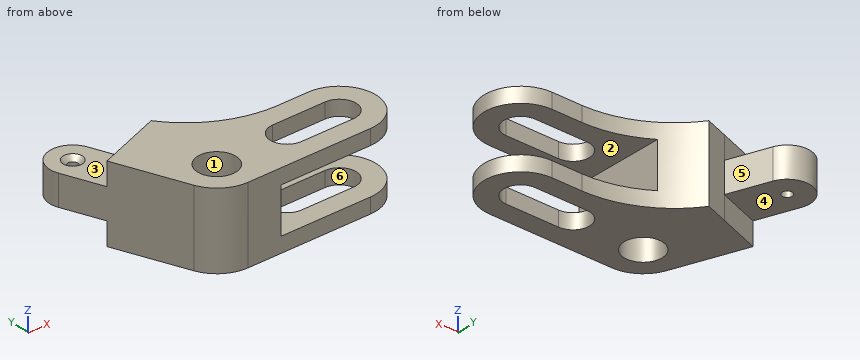
```python
from build123d import *

# Parameters (mm, degrees)
SKETCH1_R                                       = 12.5
SKETCH1_R_2                                     = 3
BOSS_EXTRUDE1_DEPTH                             = 25
SKETCH2_W                                       = 15
SKETCH2_H                                       = 43
CUT_EXTRUDE1_DEPTH                              = 50
CUT_EXTRUDE2_DEPTH                              = 125.934480099
CUT_EXTRUDE2_DEPTH_BACK                         = 125.934480099
SKETCH4_W                                       = 100
SKETCH4_H                                       = 30
CSK_FOR_M6_FLAT_HEAD_MACHINE_SCREW1_D           = 6.6
CSK_FOR_M6_FLAT_HEAD_MACHINE_SCREW1_CSINK_D     = 12.6
CSK_FOR_M6_FLAT_HEAD_MACHINE_SCREW1_CSINK_ANGLE = 90


with BuildPart() as part:
    # Sketch1 → Boss-Extrude1 (new, symmetric)
    with BuildSketch(Plane.XY):
        with BuildLine():
            Line((0, -24), (82, -24))
            ThreePointArc((82, -24), (106, 0), (82, 24))
            Line((82, 24), (62, 24))
            ThreePointArc((62, 24), (29.043180304, 32.086461832), (3.572230491, 54.509074192))
            Line((3.572230491, 54.509074192), (-11.462851442, 49.036751899))
            Line((-11.462851442, 49.036751899), (-21.039415455, 75.348145281))
            ThreePointArc((-21.039415455, 75.348145281), (-40.265106916, 84.313232443), (-49.230194078, 65.087540981))
            Line((-49.230194078, 65.087540981), (-39.653630065, 38.776147599))
            Line((-39.653630065, 38.776147599), (-22.552622899, -8.20848344))
            ThreePointArc((-22.552622899, -8.20848344), (-13.765834472, -19.659649063), (0, -24))
        make_face()
        Circle(SKETCH1_R, mode=Mode.SUBTRACT)
        with Locations((-35.134804766, 70.217843131)):
            Circle(SKETCH1_R_2, mode=Mode.SUBTRACT)
        with BuildLine():
            Line((47, 11), (82, 11))
            ThreePointArc((82, 11), (93, 0), (82, -11))
            Line((82, -11), (47, -11))
            ThreePointArc((47, -11), (36, 0), (47, 11))
        make_face(mode=Mode.SUBTRACT)
    extrude(amount=BOSS_EXTRUDE1_DEPTH, both=True)

    # Sketch2 → Cut-Extrude1 (cut)
    with BuildSketch(Plane(origin=(5.638155725, 2.05212086, 0), x_dir=(0, 0, -1), z_dir=(0.9396926207859104, 0.3420201433256632, 0))):
        with Locations((-17.5, 71.5)):
            Rectangle(SKETCH2_W, SKETCH2_H)
        with Locations((17.5, 71.5)):
            Rectangle(SKETCH2_W, SKETCH2_H)
    extrude(amount=-CUT_EXTRUDE1_DEPTH, mode=Mode.SUBTRACT)

    # Sketch4 → Cut-Extrude2 (cut, two sides: drawn at the far end of the back side and taken through both)
    with BuildSketch(Plane(origin=(0, 24, 0), x_dir=(1, 0, 0), z_dir=(0, 1, 0)).offset(-CUT_EXTRUDE2_DEPTH_BACK)):
        with Locations((72, 0)):
            Rectangle(SKETCH4_W, SKETCH4_H)
    extrude(amount=CUT_EXTRUDE2_DEPTH + CUT_EXTRUDE2_DEPTH_BACK, mode=Mode.SUBTRACT)

    # CSK for M6 Flat Head Machine Screw1 (through all)
    with Locations(Plane.XY.offset(10)):
        with Locations((-35.134804766, 70.217843131)):
            CounterSinkHole(CSK_FOR_M6_FLAT_HEAD_MACHINE_SCREW1_D / 2, CSK_FOR_M6_FLAT_HEAD_MACHINE_SCREW1_CSINK_D / 2, counter_sink_angle=CSK_FOR_M6_FLAT_HEAD_MACHINE_SCREW1_CSINK_ANGLE)


solid = part.part
```
The listing builds one solid part. Answer for the finished solid, in the listing's coordinates (mm). Face numbers are marked on the shaded views. A direction names the side the tool comes from. Round coordinates to 2 decimals unless told otherwise and drop trailing zeros. Write each loop counter-clockwise with the first axis right and the second up, starting at its lowest first coordinate (ties: lowest second). Pieces come first, ordered by that corner, then holes. Notation, with made-up numbers: (-4, -12) -> (7, -12) arc R12 cw to (7, 2) -> close; hole circle Ø6 at (69.25, 36). An arc over 180 degrees is marked (long way). Write item = value, one per line.
1) Which of the six approach directions +Z, -Z, +X, -X, +Y, -Y give full straight-line access (tool end or side, diameter ignored) to the marked faces 4, 5 and 6?
Check values:
face_4 = -Z, -X, +Y
face_5 = +Z, -Z, +Y
face_6 = +Z, -Z
2) Section D-D on x = 32.5 is taken. Write down the section's boundary in (y, z), plus the area to 3 significant figures.
Check values:
outline = (-24, -25) -> (30.4, -25) -> (30.4, -15) -> (-24, -15) -> close; (-24, 15) -> (30.4, 15) -> (30.4, 25) -> (-24, 25) -> close
area = 1,090 mm²
3) Section A-A on x = 77.5 is taken. Write down the section's boundary in (y, z).
Check values:
outline = (-24, -25) -> (-11, -25) -> (-11, -15) -> (-24, -15) -> close; (-24, 15) -> (-11, 15) -> (-11, 25) -> (-24, 25) -> close; (11, -25) -> (24, -25) -> (24, -15) -> (11, -15) -> close; (11, 15) -> (24, 15) -> (24, 25) -> (11, 25) -> close
4) For a pull along Z with two mould halves and no side action, classify the marked faces 1, 2 and 3 as released by +Z, released by -Z, zero draft, split by the parting line, or undercut.
Check values:
face_1 = zero draft
face_2 = undercut
face_3 = released by +Z
5) Straight lines are drawn through the part: line 1 along Z through (x, y) = (35.5, 8); line 2 along X through (y, z) = (4, -17); line 3 along Y through (x, z) = (0, 3). For each, find the intervals that lie inside material, in ascending order. Write a range as [from, to].
Check values:
line_1 = [-25, -15], [15, 25]
line_2 = [-27, -11.84], [11.84, 36.75], [92.25, 105.66]
line_3 = [-24, -12.5], [12.5, 53.21]
6) Given pin 1 (1 mm diameter, centred on x = -24, z = -11, fed in from +Y); pin 2 (12 mm diameter, centred on y = 72.5, z = 11, fed in from +X); pin 3 (5 mm diameter, centred on x = 62.5, z = 16.5, fed in from +Y); pin 4 (20 mm diameter, centred on x = 0, y = 0, fed in from -Z), each flat-ended and moving along its own axis, determine where each tip first touches the part or whether it passes through.
Check values:
pin_1 = 44.66
pin_2 = -17.85
pin_3 = 24.03
pin_4 = through
7) Section B-B on y = 4.5 is taken. Write down the section's boundary in (x, z), plus the area to 3 significant figures.
Check values:
outline = (-27.18, -25) -> (-11.66, -25) -> (-11.66, 25) -> (-27.18, 25) -> close; (11.66, -25) -> (36.96, -25) -> (36.96, -15) -> (22, -15) -> (22, 15) -> (36.96, 15) -> (36.96, 25) -> (11.66, 25) -> close; (92.04, -25) -> (105.57, -25) -> (105.57, -15) -> (92.04, -15) -> close; (92.04, 15) -> (105.57, 15) -> (105.57, 25) -> (92.04, 25) -> close
area = 1,860 mm²
8) Section C-C on z = 1.5 is taken. Write down the section's boundary in (x, y).
Check values:
outline = (-49.23, 65.09) -> (-22.55, -8.21) arc R24 ccw to (0, -24) -> (22, -24) -> (22, 36.3) arc R71.2 cw to (3.57, 54.51) -> (-11.46, 49.04) -> (-21.04, 75.35) arc R15 ccw to start; hole circle Ø6.6 at (-35.13, 70.22); hole circle Ø25 at (0, 0)
